Could you check a few things on this drawing? It's one solid part, dimensions in mm from its lowest x, y, z. A direction names the side the tool comes from. Coordinates: 2 decimals unless noted, no trailing zeros. Write each loop counter-clockwise with the first axis right and the second up, starting at its lowest first coordinate (ties: lowest second). Pieces come first, ordered by that corner, then holes. Notation, with made-up numbers: (79.25, 61) - (111.25, 61) arc R24 cw to (111.25, 92) - close; hole circle Ø1 at (5, -38.5). An arc over 180 degrees is marked (long way). Answer as a JSON object with one key per item and string values. Group by question number.
1) If we section it at B-B (z = 32.5): Write out the boundary of the cut face in (x, y).
2) If we section it at C-C (x = 52): Write out the boundary of the cut face in (y, z), plus the area to 3 significant figures.
3) Will these pins go through, and if not, where does the flat tip stop? pin 1 Ø7.5 at (x, z) = (63, 8.5) entering from -Y; pin 2 Ø12.5 at (y, z) = (30, 43) entering from +X; pin 3 Ø1 at (x, y) = (34, 31.5) entering from +Z; pin 4 Ø6 at (x, z) = (59.5, 30) entering from -Y.
4) Please list where these lines run through material, in increasing order: line 1 along X through (y, z) = (4.5, 18); line 2 along Z through (x, y) = (35, 41); line 3 along Y through (x, z) = (38.5, 21).
5) If we section it at A-A (y = 29): Write out the boundary of the cut face in (x, z), plus the area to 3 significant figures.
6) If we section it at D-D (y = 23): Write out the boundary of the cut face in (x, z).
7) On a 3-axis mill with a long thin cutter (end or side, diameter ignored), from which of +Z, -Z, +X, -X, +Y, -Y can I reach the whole of each face in a straight line? I mean the marked faces 1, 2, 3 and 4. Say none if no direction works.
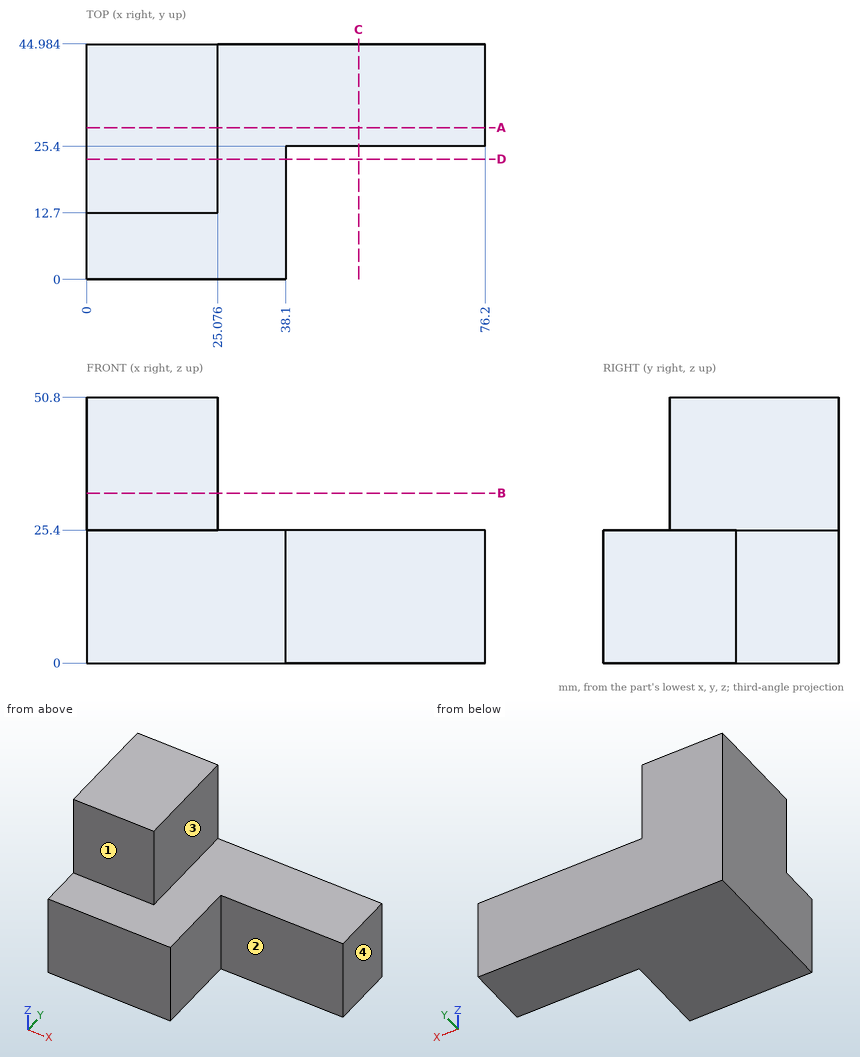
Here are the results:
{
 "1": {"outline": "(0, 12.7) - (25.08, 12.7) - (25.08, 44.98) - (0, 44.98) - close"},
 "2": {"outline": "(25.4, 0) - (44.98, 0) - (44.98, 25.4) - (25.4, 25.4) - close", "area": "497 mm²"},
 "3": {"pin 1": "stops at y = 25.4", "pin 2": "stops at x = 25.08", "pin 3": "stops at z = 25.4", "pin 4": "passes through"},
 "4": {"line 1": "x = 0 to 38.1", "line 2": "z = 0 to 25.4", "line 3": "y = 25.4 to 44.98"},
 "5": {"outline": "(0, 0) - (76.2, 0) - (76.2, 25.4) - (25.08, 25.4) - (25.08, 50.8) - (0, 50.8) - close", "area": "2,570 mm²"},
 "6": {"outline": "(0, 0) - (38.1, 0) - (38.1, 25.4) - (25.08, 25.4) - (25.08, 50.8) - (0, 50.8) - close"},
 "7": {"face 1": "+Z, +X, -X, -Y", "face 2": "+Z, -Z, +X, -Y", "face 3": "+Z, +X, +Y, -Y", "face 4": "+Z, -Z, +X, +Y, -Y"}
}
